For this review, take the finished solid that the model builds, in its own axes (mm). A direction names the side the tool comes from. Coordinates: 2 decimals unless noted, no trailing zeros. Loops run counter-clockwise (first coordinate to the right, second up) from the corner with the lowest first, then second, coordinate; pieces in that order, holes last. Notation, with made-up numbers: M -14,57 L 30,57 A28 cw 30,88 Z; hole C 57,21 d9. An arc over 180 degrees is marked long. Write item = value, one per line.
from build123d import *

# Parameters (mm, degrees)
F1_DEPTH = 0.25


with BuildPart() as f1:
    # F0 (on Right) → F1 (new body, symmetric)
    with BuildSketch(Plane.YZ):
        Polygon((1, -39.3), (1.7, -40), (6.7, -40), (6.7, -27.5), (8.5, -22), (0, 0), (0, -21.8), (1, -27.5), align=None)
        with BuildLine():
            ThreePointArc((5.15, -35), (3.85, -36.3), (2.55, -35))
            Line((2.55, -35), (2.55, -31))
            ThreePointArc((2.55, -31), (3.85, -29.7), (5.15, -31))
            Line((5.15, -31), (5.15, -35))
        make_face(mode=Mode.SUBTRACT)
    extrude(amount=F1_DEPTH, both=True)


solid = f1.part
Q1. Add section B-B (y = 4.75). Write out the cut boundary in (x, z), and give its area (3 significant figures).
Solved:
outline = M -0.25,-40 L 0.25,-40 L 0.25,-35.94 L -0.25,-35.94 Z; M -0.25,-30.06 L 0.25,-30.06 L 0.25,-12.29 L -0.25,-12.29 Z
area = 10.9 mm²
Q2. Add section A-A (x = -0.1). Write out the cut boundary in (y, z).
Solved:
outline = M 0,-21.8 L 1,-27.5 L 1,-39.3 L 1.7,-40 L 6.7,-40 L 6.7,-27.5 L 8.5,-22 L 0,0 Z; hole M 2.55,-35 A1.3 ccw 5.15,-35 L 5.15,-31 A1.3 ccw 2.55,-31 Z
Q3. For line 1 along Y through (x, z) = (0.1, -29); line 2 along Y through (x, z) = (0.2, -22.5), list the stretches that pass through material, from the lowest coordinate up.
Solved:
line_1 = 1 to 6.7
line_2 = 0.12 to 8.34
Q4. Add section D-D (y = 3.25). Write out the cut boundary in (x, z), and give its area (3 significant figures).
Solved:
outline = M -0.25,-40 L 0.25,-40 L 0.25,-36.15 L -0.25,-36.15 Z; M -0.25,-29.85 L 0.25,-29.85 L 0.25,-8.41 L -0.25,-8.41 Z
area = 12.6 mm²
Q5. Draft analysis for pull direction Z (two halves, no side actions). For faces 1 (the face through (0.004, 0.493, -24.61)), 2 (the face through (0, 4.31, -11.15)), 3 (the face through (0, 3.9, -36.3)), 4 (the face through (-0.25, 3, -24)), state which applies: +Z half, -Z half, draft (parallel to the pull), parting line (faces both ways), or undercut.
Solved:
face_1 = -Z half
face_2 = +Z half
face_3 = undercut
face_4 = draft
Q6. Machinability: for faces 5 (the face through (0, 3.8, -29.7)), 6 (the face through (0.25, 3, -24)), which of the approach directions +Z, -Z, +X, -X, +Y, -Y give a long, thin tool a straight path to every point of the face, cutting with its end or side? Answer none if there is none.
Solved:
face_5 = +X, -X
face_6 = +Z, -Z, +X, +Y, -Y
Q7. Add section C-C (z = -28). Write out the cut boundary in (x, y), and give its area (3 significant figures).
Solved:
outline = M -0.25,1 L 0.25,1 L 0.25,6.7 L -0.25,6.7 Z
area = 2.85 mm²
